```python
from build123d import *

# Parameters (mm, degrees)
SKETCH1_W                    = 110
SKETCH1_H                    = 100
BASE_FLANGE1_DEPTH           = 1.5
EDGE_FLANGE1_STRIP_W         = 9
EDGE_FLANGE1_STRIP_H         = 1.5
EDGE_FLANGE1_STRIP_CUT_DEPTH = 110
EDGE_FLANGE1_DEPTH           = 110
EDGE_FLANGE1_FLAT_DEPTH      = 1.5
EDGE_FLANGE2_DEPTH           = 31.5
F_4_0_4_DIAMETER_HOLE1_D     = 4
EDGE_FLANGE3_DEPTH           = 94
EDGE_FLANGE3_BEND_DEPTH      = 94
F_12_0_12_DIAMETER_HOLE1_D   = 12
EDGE_FLANGE4_STRIP_W         = 9
EDGE_FLANGE4_STRIP_H         = 1.5
EDGE_FLANGE4_STRIP_CUT_DEPTH = 40
EDGE_FLANGE4_DEPTH           = 40


# Sheet-metal steps are written as plain solids
with BuildPart() as part:
    # Sketch1 → Base-Flange1 (new body)
    with BuildSketch(Plane(origin=(0, 0, 0), x_dir=(1, 0, 0), z_dir=(0, 1, 0))):
        with Locations((12, 0)):
            Rectangle(SKETCH1_W, SKETCH1_H)
        with BuildLine():
            Line((24.494897428, -25), (39.494897428, -25))
            Line((39.494897428, -25), (39.494897428, -20))
            Line((39.494897428, -20), (31.494897428, -20))
            Line((31.494897428, -20), (31.494897428, 20))
            Line((31.494897428, 20), (39.494897428, 20))
            Line((39.494897428, 20), (39.494897428, 25))
            Line((39.494897428, 25), (24.494897428, 25))
            ThreePointArc((24.494897428, 25), (-35, 0), (24.494897428, -25))
        make_face(mode=Mode.SUBTRACT)
    extrude(amount=-BASE_FLANGE1_DEPTH)

    # Edge-Flange1 strip (across the edge) → Edge-Flange1 strip cut (cut)
    with BuildSketch(Plane(origin=(67, -1.5, 50), x_dir=(0, 0, -1), z_dir=(-1, 0, 0))):
        with Locations((-1.5, -0.75)):
            Rectangle(EDGE_FLANGE1_STRIP_W, EDGE_FLANGE1_STRIP_H)
    edge_flange1_strip_cut = extrude(amount=EDGE_FLANGE1_STRIP_CUT_DEPTH, mode=Mode.SUBTRACT)

    # Edge-Flange1 bend section (across the edge) → Edge-Flange1 (add)
    with BuildSketch(Plane(origin=(67, -1.5, 50), x_dir=(0, 0, -1), z_dir=(-1, 0, 0))):
        with BuildLine():
            Line((0, 1.5), (1.5, 1.5))
            ThreePointArc((1.5, 1.5), (1.939339828, 0.439339828), (3, 0))
            Line((3, 0), (3, -1.5))
            ThreePointArc((3, -1.5), (0.878679656, -0.621320344), (0, 1.5))
        make_face()
    edge_flange1 = extrude(amount=EDGE_FLANGE1_DEPTH)

    # Edge-Flange1 profile (on flange) → Edge-Flange1 flat (add)
    with BuildSketch(Plane(origin=(0, -1.5, 50), x_dir=(1, 0, 0), z_dir=(0, 0, -1))):
        Polygon((-43, 1.5), (67, 1.5), (67, 40), (7, 4.5), (-43, 4.5), align=None)
    edge_flange1_flat = extrude(amount=EDGE_FLANGE1_FLAT_DEPTH)

    # Edge-Flange2 section (across the edge) → Edge-Flange2 (add)
    with BuildSketch(Plane(origin=(68.5, -10, 48.5), x_dir=(-1, 0, 0), z_dir=(0, -1, 0))):
        with BuildLine():
            Line((-1.5, 1.5), (-1.5, 8.5))
            Line((-1.5, 8.5), (0, 8.5))
            Line((0, 8.5), (0, 1.5))
            ThreePointArc((0, 1.5), (0.439339828, 0.439339828), (1.5, 0))
            Line((1.5, 0), (1.5, -1.5))
            ThreePointArc((1.5, -1.5), (-0.621320344, -0.621320344), (-1.5, 1.5))
        make_face()
    edge_flange2 = extrude(amount=EDGE_FLANGE2_DEPTH)

    # Ø4.0 (4) Diameter Hole1 (through all)
    with Locations(Plane(origin=(70, 0, 0), x_dir=(0, 0, -1), z_dir=(1, 0, 0))):
        with Locations((-43, -17.5), (-43, -35.5)):
            f_4_0_4_diameter_hole1 = Hole(F_4_0_4_DIAMETER_HOLE1_D / 2)

    # Mirror1: Edge-Flange1 strip cut, Edge-Flange1, Edge-Flange1 flat, Edge-Flange2, Ø4.0 (4) Diameter Hole1 across plane
    add(edge_flange1_strip_cut.mirror(Plane.XY), mode=Mode.SUBTRACT)
    add(edge_flange1.mirror(Plane.XY))
    add(edge_flange1_flat.mirror(Plane.XY))
    add(edge_flange2.mirror(Plane.XY))
    add(f_4_0_4_diameter_hole1.mirror(Plane.XY), mode=Mode.SUBTRACT)

    # Edge-Flange3 section (across the edge) → Edge-Flange3 (add)
    with BuildSketch(Plane(origin=(68.5, -1.5, -47), x_dir=(-1, 0, 0), z_dir=(0, 0, 1))):
        with BuildLine():
            Line((-1.5, 1.5), (-1.5, 4.5))
            Line((-1.5, 4.5), (0, 4.5))
            Line((0, 4.5), (0, 1.5))
            ThreePointArc((0, 1.5), (0.439339828, 0.439339828), (1.5, 0))
            Line((1.5, 0), (1.5, -1.5))
            ThreePointArc((1.5, -1.5), (-0.621320344, -0.621320344), (-1.5, 1.5))
        make_face()
    extrude(amount=EDGE_FLANGE3_DEPTH)

    # Edge-Flange3 section 2 (across the edge) → Edge-Flange3 bend (add)
    with BuildSketch(Plane(origin=(-44.5, -1.5, 47), x_dir=(1, 0, 0), z_dir=(0, 0, -1))):
        with BuildLine():
            Line((-1.5, 1.5), (-1.5, 4.5))
            Line((-1.5, 4.5), (0, 4.5))
            Line((0, 4.5), (0, 1.5))
            ThreePointArc((0, 1.5), (0.439339828, 0.439339828), (1.5, 0))
            Line((1.5, 0), (1.5, -1.5))
            ThreePointArc((1.5, -1.5), (-0.621320344, -0.621320344), (-1.5, 1.5))
        make_face()
    extrude(amount=EDGE_FLANGE3_BEND_DEPTH)

    # Ø12.0 (12) Diameter Hole1 (through all)
    with Locations(Plane(origin=(0, 0, 0), x_dir=(1, 0, 0), z_dir=(0, 1, 0))):
        with Locations((54, 34), (54, -34)):
            Hole(F_12_0_12_DIAMETER_HOLE1_D / 2)

    # Edge-Flange4 strip (across the edge) → Edge-Flange4 strip cut (cut)
    with BuildSketch(Plane(origin=(31.494897428, 0, -20), x_dir=(1, 0, 0), z_dir=(0, 0, 1))):
        with Locations((-1.5, -0.75)):
            Rectangle(EDGE_FLANGE4_STRIP_W, EDGE_FLANGE4_STRIP_H)
    extrude(amount=EDGE_FLANGE4_STRIP_CUT_DEPTH, mode=Mode.SUBTRACT)

    # Edge-Flange4 section (across the edge) → Edge-Flange4 (add)
    with BuildSketch(Plane(origin=(31.494897428, 0, -20), x_dir=(1, 0, 0), z_dir=(0, 0, 1))):
        with BuildLine():
            Line((0, 1.5), (0, 6.5))
            Line((0, 6.5), (1.5, 6.5))
            Line((1.5, 6.5), (1.5, 1.5))
            ThreePointArc((1.5, 1.5), (1.939339828, 0.439339828), (3, 0))
            Line((3, 0), (3, -1.5))
            ThreePointArc((3, -1.5), (0.878679656, -0.621320344), (0, 1.5))
        make_face()
    extrude(amount=EDGE_FLANGE4_DEPTH)


solid = part.part
```
For this review, take the finished solid that the model builds, in its own axes (mm). A direction names the side the tool comes from. Give positions to 0.01 mm unless a question says otherwise; leave off trailing zeros. Write each loop counter-clockwise with the first axis right and the second up, starting at its lowest first coordinate (ties: lowest second). Pieces come first, ordered by that corner, then holes.
Item 1: Machinability: for faces 4 (the face through (36, -1.5, -1)), 5 (the face through (69, -10, 45)), 6 (the face through (40, -15, -48.5)), 7 (the face through (-44.5, -5, 1)), 8 (the face through (33.8, -0.1, -20)), which of the approach directions +Z, -Z, +X, -X, +Y, -Y give a long, thin tool a straight path to every point of the face, cutting with its end or side? Answer none if there is none.
Item 2: Insertion check: P1, Ø1.5, axis at y = -3.5, z = 48, coming from the -X side; P2, Ø4, axis at x = 30.5, z = -24, coming from the +Y side; P3, Ø0.9, axis at x = -44.5, y = -4, coming from the -Z side. Each pin has a flat end and moves straight along its axis. Give the tip position at first contact, or say it passes through.
Item 3: Take a section at B-B (z = 0). Give the boundary of the cut face in (x, y).
Item 4: Take a section at A-A (z = -43). Give the boundary of the cut face in (x, y), and give its area (3 significant figures).
Item 5: Take a section at D-D (x = 5). Give the boundary of the cut face in (y, z), and give its area (3 significant figures).
Item 6: Take a section at C-C (y = -17.5). Give the boundary of the cut face in (x, z).
Item 7: The part is to be moulded in two halves that separate along Z. For faces 1 (the face through (40, -15, -50)), 2 (the face through (-43, -3, 49)), 3 (the face through (-34.98, -0.74, -1.15)), say which applies: +Z half, -Z half, draft (parallel to the pull), parting line (faces both ways), or undercut.
Item 8: Wall thickness on probe 1 along Z at (x, y) = (-35.5, -5); probe 2 along Y at (x, z) = (69.7, 43); probe 3 along Z at (x, y) = (54, -0.6): over which ranges is each line inside the solid? List them lowest first.
Established:
1. face 4: -Y
1. face 5: +Z, -Z, +X
1. face 6: -X, -Y
1. face 7: +Z, -Z, -Y
1. face 8: +Y, -Y
2. P1: stops at x = -43
2. P2: stops at y = 0
2. P3: stops at z = -47
3. outline: (-46, -6) - (-44.5, -6) - (-44.5, -3) arc R1.5 cw to (-43, -1.5) - (-35, -1.5) - (-35, 0) - (-43, 0) arc R3 ccw to (-46, -3) - close; (31.49, 1.5) arc R3 ccw to (34.49, -1.5) - (67, -1.5) arc R1.5 cw to (68.5, -3) - (68.5, -6) - (70, -6) - (70, -3) arc R3 ccw to (67, 0) - (34.49, 0) arc R1.5 cw to (32.99, 1.5) - (32.99, 6.5) - (31.49, 6.5) - close
4. outline: (-46, -6) - (-44.5, -6) - (-44.5, -3) arc R1.5 cw to (-43, -1.5) - (67, -1.5) arc R1.5 cw to (68.5, -3) - (68.5, -6) - (70, -6) - (70, -3) arc R3 ccw to (67, 0) - (-43, 0) arc R3 ccw to (-46, -3) - close; (68.5, -41.5) - (70, -41.5) - (70, -37.5) - (68.5, -37.5) - close; (68.5, -33.5) - (70, -33.5) - (70, -19.5) - (68.5, -19.5) - close; (68.5, -15.5) - (70, -15.5) - (70, -10) - (68.5, -10) - close
4. area: 220 mm2
5. outline: (-6, -50) - (-3, -50) arc R3 ccw to (0, -47) - (0, -34.64) - (-1.5, -34.64) - (-1.5, -47) arc R1.5 cw to (-3, -48.5) - (-6, -48.5) - close; (-6, 48.5) - (-3, 48.5) arc R1.5 cw to (-1.5, 47) - (-1.5, 34.64) - (0, 34.64) - (0, 47) arc R3 ccw to (-3, 50) - (-6, 50) - close
5. area: 56.7 mm2
6. outline: (26.44, -50) - (67, -50) arc R3 ccw to (70, -47) - (70, -45) - (68.5, -45) - (68.5, -47) arc R1.5 cw to (67, -48.5) - (26.44, -48.5) - close; (26.44, 48.5) - (67, 48.5) arc R1.5 cw to (68.5, 47) - (68.5, 45) - (70, 45) - (70, 47) arc R3 ccw to (67, 50) - (26.44, 50) - close; (68.5, -41) - (70, -41) - (70, -40) - (68.5, -40) - close; (68.5, 40) - (70, 40) - (70, 41) - (68.5, 41) - close
7. face 1: -Z half
7. face 2: draft
7. face 3: undercut
8. probe 1: z = -50 to -48.5, 48.5 to 50
8. probe 2: y = -41.5 to -37.5, -33.5 to -19.5, -15.5 to -10, -6 to -1.69
8. probe 3: z = -48.8 to -40, -28 to 28, 40 to 48.8
